from build123d import *

# Parameters (mm, degrees)
F0_R     = 2.25
F1_DEPTH = 1.5
F2_R     = 1


with BuildPart() as f1:
    # F0 (on Top) → F1 (new body)
    with BuildSketch(Plane.XY):
        with BuildLine():
            Line((-19.346866, -5), (69, -5))
            ThreePointArc((69, -5), (71.12132, -4.12132), (72, -2))
            Line((72, -2), (72, 2))
            ThreePointArc((72, 2), (71.12132, 4.12132), (69, 5))
            Line((69, 5), (-69, 5))
            ThreePointArc((-69, 5), (-71.12132, 4.12132), (-72, 2))
            Line((-72, 2), (-72, -2))
            ThreePointArc((-72, -2), (-71.12132, -4.12132), (-69, -5))
            Line((-69, -5), (-26.346866, -5))
            Line((-26.346866, -5), (-26.346866, 2))
            Line((-26.346866, 2), (-25.846866, 2))
            Line((-25.846866, 2), (-19.846866, 2))
            Line((-19.846866, 2), (-19.346866, 2))
            Line((-19.346866, 2), (-19.346866, -5))
        make_face()
        with Locations((-66.75, 0)):
            Circle(F0_R, mode=Mode.SUBTRACT)
        with BuildLine():
            ThreePointArc((-4, -2.25), (-4.292893, -2.957107), (-5, -3.25))
            Line((-5, -3.25), (-6, -3.25))
            ThreePointArc((-6, -3.25), (-6.707107, -2.957107), (-7, -2.25))
            Line((-7, -2.25), (-7, 2.25))
            ThreePointArc((-7, 2.25), (-6.707107, 2.957107), (-6, 3.25))
            Line((-6, 3.25), (-5, 3.25))
            ThreePointArc((-5, 3.25), (-4.292893, 2.957107), (-4, 2.25))
            Line((-4, 2.25), (-4, -2.25))
        make_face(mode=Mode.SUBTRACT)
        with BuildLine():
            ThreePointArc((4, -3.25), (3.292893, -2.957107), (3, -2.25))
            Line((3, -2.25), (3, 2.25))
            ThreePointArc((3, 2.25), (3.292893, 2.957107), (4, 3.25))
            Line((4, 3.25), (5, 3.25))
            ThreePointArc((5, 3.25), (5.707107, 2.957107), (6, 2.25))
            Line((6, 2.25), (6, -2.25))
            ThreePointArc((6, -2.25), (5.707107, -2.957107), (5, -3.25))
            Line((5, -3.25), (4, -3.25))
        make_face(mode=Mode.SUBTRACT)
        with BuildLine():
            ThreePointArc((14, -3.25), (13.292893, -2.957107), (13, -2.25))
            Line((13, -2.25), (13, 2.25))
            ThreePointArc((13, 2.25), (13.292893, 2.957107), (14, 3.25))
            Line((14, 3.25), (15, 3.25))
            ThreePointArc((15, 3.25), (15.707107, 2.957107), (16, 2.25))
            Line((16, 2.25), (16, -2.25))
            ThreePointArc((16, -2.25), (15.707107, -2.957107), (15, -3.25))
            Line((15, -3.25), (14, -3.25))
        make_face(mode=Mode.SUBTRACT)
        with BuildLine():
            ThreePointArc((24, -3.25), (23.292893, -2.957107), (23, -2.25))
            Line((23, -2.25), (23, 2.25))
            ThreePointArc((23, 2.25), (23.292893, 2.957107), (24, 3.25))
            Line((24, 3.25), (25, 3.25))
            ThreePointArc((25, 3.25), (25.707107, 2.957107), (26, 2.25))
            Line((26, 2.25), (26, -2.25))
            ThreePointArc((26, -2.25), (25.707107, -2.957107), (25, -3.25))
            Line((25, -3.25), (24, -3.25))
        make_face(mode=Mode.SUBTRACT)
        with BuildLine():
            ThreePointArc((34, -3.25), (33.292893, -2.957107), (33, -2.25))
            Line((33, -2.25), (33, 2.25))
            ThreePointArc((33, 2.25), (33.292893, 2.957107), (34, 3.25))
            Line((34, 3.25), (35, 3.25))
            ThreePointArc((35, 3.25), (35.707107, 2.957107), (36, 2.25))
            Line((36, 2.25), (36, -2.25))
            ThreePointArc((36, -2.25), (35.707107, -2.957107), (35, -3.25))
            Line((35, -3.25), (34, -3.25))
        make_face(mode=Mode.SUBTRACT)
        with BuildLine():
            ThreePointArc((44, -3.25), (43.292893, -2.957107), (43, -2.25))
            Line((43, -2.25), (43, 2.25))
            ThreePointArc((43, 2.25), (43.292893, 2.957107), (44, 3.25))
            Line((44, 3.25), (45, 3.25))
            ThreePointArc((45, 3.25), (45.707107, 2.957107), (46, 2.25))
            Line((46, 2.25), (46, -2.25))
            ThreePointArc((46, -2.25), (45.707107, -2.957107), (45, -3.25))
            Line((45, -3.25), (44, -3.25))
        make_face(mode=Mode.SUBTRACT)
        with BuildLine():
            ThreePointArc((54, -3.25), (53.292893, -2.957107), (53, -2.25))
            Line((53, -2.25), (53, 2.25))
            ThreePointArc((53, 2.25), (53.292893, 2.957107), (54, 3.25))
            Line((54, 3.25), (55, 3.25))
            ThreePointArc((55, 3.25), (55.707107, 2.957107), (56, 2.25))
            Line((56, 2.25), (56, -2.25))
            ThreePointArc((56, -2.25), (55.707107, -2.957107), (55, -3.25))
            Line((55, -3.25), (54, -3.25))
        make_face(mode=Mode.SUBTRACT)
        with BuildLine():
            ThreePointArc((64, -3.25), (63.292893, -2.957107), (63, -2.25))
            Line((63, -2.25), (63, 2.25))
            ThreePointArc((63, 2.25), (63.292893, 2.957107), (64, 3.25))
            Line((64, 3.25), (65, 3.25))
            ThreePointArc((65, 3.25), (65.707107, 2.957107), (66, 2.25))
            Line((66, 2.25), (66, -2.25))
            ThreePointArc((66, -2.25), (65.707107, -2.957107), (65, -3.25))
            Line((65, -3.25), (64, -3.25))
        make_face(mode=Mode.SUBTRACT)
        Polygon((-19.846866, -8), (-19.846866, -5), (-19.846866, 2), (-25.846866, 2), (-25.846866, -5), (-25.846866, -8), align=None)
    extrude(amount=F1_DEPTH)

    # F2
    f2_edges = [f1.edges().sort_by_distance(p)[0] for p in [
        (-25.846866, -8, 0.75),
        (-19.846866, -8, 0.75),
    ]]
    fillet(f2_edges, radius=F2_R)


solid = f1.part
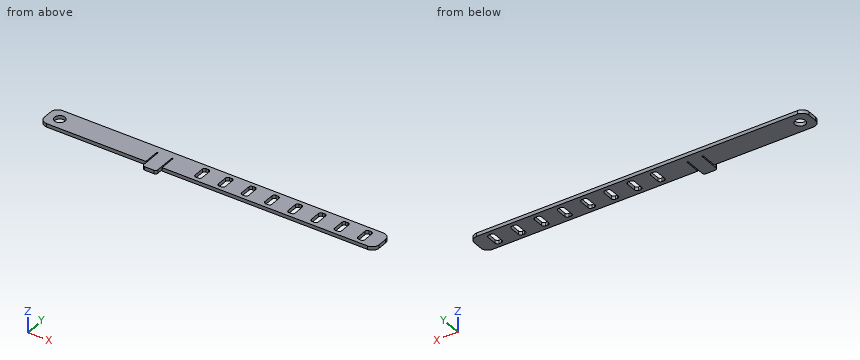
The model under review builds one solid part; all positions refer to its coordinate system, in mm. Give positions to 0.01 mm unless a question says otherwise; leave off trailing zeros. Write each loop counter-clockwise with the first axis right and the second up, starting at its lowest first coordinate (ties: lowest second). Pieces come first, ordered by that corner, then holes.
1. Wall thickness on L1, parallel to Y at x = -66.75, z = 0.7; L2, parallel to Y at x = 45, z = 1.35; L3, parallel to Y at x = 61, z = 0.7: over which ranges is each line inside the solid? List them lowest first.
2. For P1, Ø0.5, axis at x = 14.5, z = 0.5, coming from the -Y side, flat-tipped, find the tip position at first contact; note if it passes through.
3. Add section A-A, the plane x = -66.75. Write out the cut boundary in (y, z).
4. Add section D-D, the plane x = -17. Write out the cut boundary in (y, z).
5. Add section B-B, the plane y = 0. Count the separate pieces of the cut face and the enclosed holes in it, plus the area to 3 significant figures.
Worked answers:
1. L1: y = -5 to -2.25, 2.25 to 5
1. L2: y = -5 to -3.25, 3.25 to 5
1. L3: y = -5 to 5
2. P1: stops at y = -5
3. outline: (-5, 0) - (-2.25, 0) - (-2.25, 1.5) - (-5, 1.5) - close; (2.25, 0) - (5, 0) - (5, 1.5) - (2.25, 1.5) - close
4. outline: (-5, 0) - (5, 0) - (5, 1.5) - (-5, 1.5) - close
5. separate pieces: 12
5. enclosed holes: 0
5. area: 172 mm2
